The figure shows three views and two pictorial views of one solid part (mm, origin at its lowest corner). Answer the questions. A direction names the side the tool comes from. Round coordinates to 2 decimals unless told otherwise and drop trailing zeros. Order: outer loops, then holes, each group sorted by start corner. A loop starts at its lowest first (then second) coordinate and runs counter-clockwise, first axis right, second up. Notation, with made-up numbers: (4, 38.25) - (51, 38.25) arc R32 cw to (51, 64.25) - close; hole circle Ø3 at (18, 47.25). An arc over 180 degrees is marked (long way). Write item = value, one per line.
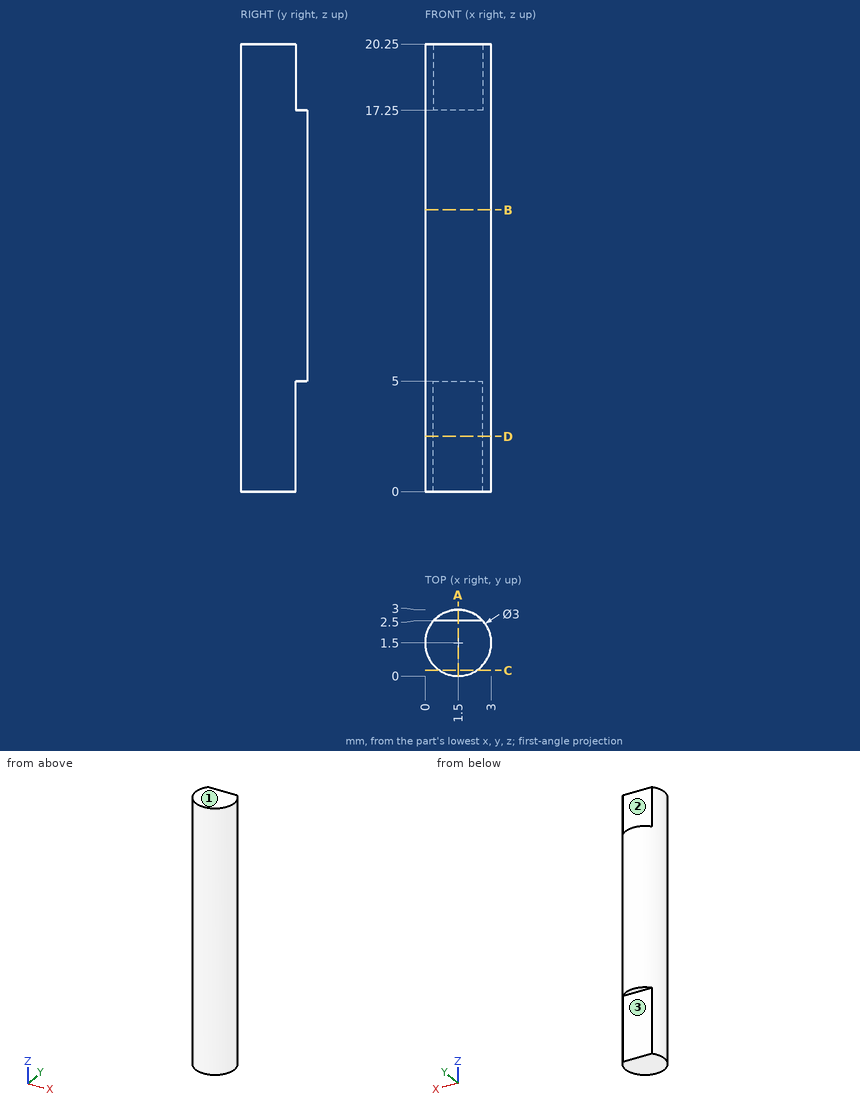
Q1. Flat-ended cylindrical pins translate along their axes: P1, Ø1, axis at x = 2.5, z = 8, coming from the +Y side; P2, Ø0.7, axis at x = 2, z = 3, coming from the +Y side. Find the tip coordinate at first contact, or state that the pin passes through.
Model answer:
P1 = 2.91
P2 = 2.5
Q2. For the marked faces 1, 2 and 3, determine the directions among +Z, -Z, +X, -X, +Y, -Y from which every point of the face is accessible in a straight line to the end or side of a thin tool.
Model answer:
face_1 = +Z, +X, -X, +Y, -Y
face_2 = +Z, +X, -X, +Y
face_3 = -Z, +X, -X, +Y
Q3. Find the intervals of material crossed by line 1 (X direction, y = 1.4, z = 8.25); line 2 (Y direction, x = 2.5, z = 18.5); line 3 (X direction, y = 0.5, z = 1.25), in increasing order. Write a range as from..to.
Model answer:
line_1 = 0..3
line_2 = 0.38..2.5
line_3 = 0.38..2.62
Q4. Section D-D on z = 2.5 is taken. Determine the outline of the cut face in (x, y), then the cut area to 3 significant figures.
Model answer:
outline = (0.38, 2.5) arc R1.5 ccw (long way) to (2.62, 2.5) - close
area = 6.29 mm^2
Q5. Section C-C on y = 0.25 is taken. Determine the outline of the cut face in (x, z).
Model answer:
outline = (0.67, 0) - (2.33, 0) - (2.33, 20.25) - (0.67, 20.25) - close
Q6. Section B-B on z = 12.75 is taken. Determine the outline of the cut face in (x, y), then the cut area to 3 significant figures.
Model answer:
outline = circle Ø3 at (1.5, 1.5)
area = 7.07 mm^2
Q7. Section A-A on x = 1.5 is taken. Determine the outline of the cut face in (y, z), then the cut area to 4 significant figures.
Model answer:
outline = (0, 0) - (2.5, 0) - (2.5, 5) - (3, 5) - (3, 17.25) - (2.5, 17.25) - (2.5, 20.25) - (0, 20.25) - close
area = 56.75 mm^2
